```python
from build123d import *

# Parameters (mm, degrees)
SKETCH1_W           = 80
SKETCH1_H           = 80
BOSS_EXTRUDE1_DEPTH = 1.5875
SKETCH2_OUTSIDE_W   = 104.636
SKETCH2_OUTSIDE_H   = 104.636
CUT_EXTRUDE1_DEPTH  = 57.657573413
SKETCH3_W           = 80
SKETCH3_H           = 6.153846154
BOSS_EXTRUDE2_DEPTH = 3.175


with BuildPart() as part:
    # Sketch1 → Boss-Extrude1 (new, symmetric)
    with BuildSketch(Plane(origin=(0, 0, 0), x_dir=(1, 0, 0), z_dir=(0, 1, 0))):
        Rectangle(SKETCH1_W, SKETCH1_H)
    extrude(amount=BOSS_EXTRUDE1_DEPTH, both=True)

    # Sketch2 outside → Cut-Extrude1 (cut, through all)
    with BuildSketch(Plane(origin=(0, 1.5875, 0), x_dir=(1, 0, 0), z_dir=(0, 1, 0))):
        Rectangle(SKETCH2_OUTSIDE_W, SKETCH2_OUTSIDE_H)
        Polygon((-40, 40), (-40, 33.846153846), (-36.82, 33.846153846), (-36.82, 27.692307692), (-40, 27.692307692), (-40, 21.538461538), (-36.82, 21.538461538), (-36.82, 15.384615385), (-40, 15.384615385), (-40, 9.230769231), (-36.82, 9.230769231), (-36.82, 3.076923077), (-40, 3.076923077), (-40, -3.076923077), (-36.82, -3.076923077), (-36.82, -9.230769231), (-40, -9.230769231), (-40, -15.384615385), (-36.82, -15.384615385), (-36.82, -21.538461538), (-40, -21.538461538), (-40, -27.692307692), (-36.82, -27.692307692), (-36.82, -33.846153846), (-40, -33.846153846), (-40, -40), (-33.846153846, -40), (-33.846153846, -36.82), (-27.692307692, -36.82), (-27.692307692, -40), (-21.538461538, -40), (-21.538461538, -36.82), (-15.384615385, -36.82), (-15.384615385, -40), (-9.230769231, -40), (-9.230769231, -36.82), (-3.076923077, -36.82), (-3.076923077, -40), (3.076923077, -40), (3.076923077, -36.82), (9.230769231, -36.82), (9.230769231, -40), (15.384615385, -40), (15.384615385, -36.82), (21.538461538, -36.82), (21.538461538, -40), (27.692307692, -40), (27.692307692, -36.82), (33.846153846, -36.82), (33.846153846, -40), (40, -40), (40, -33.846153846), (36.82, -33.846153846), (36.82, -27.692307692), (40, -27.692307692), (40, -21.538461538), (36.82, -21.538461538), (36.82, -15.384615385), (40, -15.384615385), (40, -9.230769231), (36.82, -9.230769231), (36.82, -3.076923077), (40, -3.076923077), (40, 3.076923077), (36.82, 3.076923077), (36.82, 9.230769231), (40, 9.230769231), (40, 15.384615385), (36.82, 15.384615385), (36.82, 21.538461538), (40, 21.538461538), (40, 27.692307692), (36.82, 27.692307692), (36.82, 33.846153846), (40, 33.846153846), (40, 40), (33.846153846, 40), (33.846153846, 36.82), (27.692307692, 36.82), (27.692307692, 40), (21.538461538, 40), (21.538461538, 36.82), (15.384615385, 36.82), (15.384615385, 40), (9.230769231, 40), (9.230769231, 36.82), (3.076923077, 36.82), (3.076923077, 40), (-3.076923077, 40), (-3.076923077, 36.82), (-9.230769231, 36.82), (-9.230769231, 40), (-15.384615385, 40), (-15.384615385, 36.82), (-21.538461538, 36.82), (-21.538461538, 40), (-27.692307692, 40), (-27.692307692, 36.82), (-33.846153846, 36.82), (-33.846153846, 40), align=None, mode=Mode.SUBTRACT)
    extrude(amount=-CUT_EXTRUDE1_DEPTH, mode=Mode.SUBTRACT)

    # Sketch3 → Boss-Extrude2 (add)
    with BuildSketch(Plane(origin=(0, 1.5875, 0), x_dir=(1, 0, 0), z_dir=(0, 1, 0))):
        with Locations((0, 36.923076923)):
            Rectangle(SKETCH3_W, SKETCH3_H)
    extrude(amount=-BOSS_EXTRUDE2_DEPTH)


solid = part.part
```
Can you work these out from the model? Positions are in its coordinate system, mm. A direction names the side the tool comes from. Round coordinates to 2 decimals unless told otherwise and drop trailing zeros. Loops run counter-clockwise (first coordinate to the right, second up) from the corner with the lowest first, then second, coordinate; pieces in that order, holes last. Notation, with made-up numbers: M 52.25,-39.5 L 93.25,-39.5 A24 cw 93.25,-26.5 Z; hole C 27.25,-26 d5. An arc over 180 degrees is marked long. Answer as a JSON object with one key per item and string values. Group by question number.
Q1. Imagine slicing it at A-A, the plane z = 7. Please give me the cut outline in (x, y).
Q2. Imagine slicing it at B-B, the plane x = 7.5. Please give me the cut outline in (y, z).
Q3. Please list where these lines run through material, in increasing order: L1, parallel to Z at x = 8.5, y = 0.1; L2, parallel to X at y = -1.1, z = 29.5.
Q4. On a 3-axis mill with a long thin cutter (end or side, diameter ignored), from which of +Z, -Z, +X, -X, +Y, -Y can I reach the whole of each face in a straight line? I mean faces 1 (the flat face through (-38, 0, -21.538)), 2 (the flat face through (38, 0, 27.692)), 3 (the flat face through (40, 0, -37)), 4 (the flat face through (15.385, 0, 38)). Say none if no direction works.
Q5. We'd pull the mould along Z, two halves only. Please class faces 5 (the flat face through (21.538, 0, 38)), 6 (the flat face through (-6, 0, 36.82)), 7 (the flat face through (38, 0, -33.846)): +Z half, -Z half, draft (parallel to the pull), parting line (faces both ways), or undercut.
Findings:
{
 "1": {"outline": "M -36.82,-1.59 L 36.82,-1.59 L 36.82,1.59 L -36.82,1.59 Z"},
 "2": {"outline": "M -1.59,-40 L 1.59,-40 L 1.59,36.82 L -1.59,36.82 Z"},
 "3": {"L1": "z = -40 to 36.82", "L2": "x = -36.82 to 36.82"},
 "4": {"face 1": "-X, +Y, -Y", "face 2": "+X, +Y, -Y", "face 3": "+Z, -Z, +X, +Y, -Y", "face 4": "+Z, +Y, -Y"},
 "5": {"face 5": "draft", "face 6": "+Z half", "face 7": "undercut"}
}
